```python
from build123d import *

# Parameters (mm, degrees)
CUT_EXTRUDE1_DEPTH      = 4
CUT_EXTRUDE1_DEPTH_BACK = 4
SKETCH2_W               = 41
SKETCH2_H               = 1.5
SKETCH4_W               = 1.2295
SKETCH4_H               = 15
CUT_EXTRUDE2_DEPTH      = 8
CUT_EXTRUDE2_DEPTH_BACK = 8
SKETCH5_W               = 30
SKETCH5_H               = 3.75


with BuildPart() as part:
    # Sketch1 → Revolve1 (revolve)
    with BuildSketch(Plane(origin=(0, 0, 0), x_dir=(0, 0, -1), z_dir=(1, 0, 0)), mode=Mode.PRIVATE) as revolve1_sk:
        Polygon((-4, 8.5), (-3.5, 8), (3.5, 8), (4, 8.5), (4, 14.5), (3.5, 15), (-3.5, 15), (-4, 14.5), align=None)
    revolve(revolve1_sk.sketch.rotate(Axis((0, 0, -4), (0, 0, 1)), 270), axis=Axis((0, 0, -4), (0, 0, 1)))

    # Sketch2 → Cut-Extrude1 (cut, two sides: drawn at the far end of the back side and taken through both)
    with BuildSketch(Plane.XY.offset(-CUT_EXTRUDE1_DEPTH_BACK)):
        with Locations((-9.5, 0)):
            Rectangle(SKETCH2_W, SKETCH2_H)
    extrude(amount=CUT_EXTRUDE1_DEPTH + CUT_EXTRUDE1_DEPTH_BACK, mode=Mode.SUBTRACT)

    # Sketch3 → Cut-Revolve1 (revolve, cut)
    with BuildSketch(Plane.XY, mode=Mode.PRIVATE) as cut_revolve1_sk:
        Polygon((-11.5, -15), (-14.5, -15), (-14.5, -3), (-13.2, -3), (-13.2, 0), (-11.5, 0), align=None)
    revolve(cut_revolve1_sk.sketch.rotate(Axis((-11.5, 0, 0), (0, -1, 0)), 270), axis=Axis((-11.5, 0, 0), (0, -1, 0)), mode=Mode.SUBTRACT)

    # Sketch4 → Cut-Revolve2 (revolve, cut)
    with BuildSketch(Plane.XY, mode=Mode.PRIVATE) as cut_revolve2_sk:
        with Locations((-12.11475, 8.25)):
            Rectangle(SKETCH4_W, SKETCH4_H)
    revolve(cut_revolve2_sk.sketch.rotate(Axis((-11.5, 15.75, 0), (0, -1, 0)), 270), axis=Axis((-11.5, 15.75, 0), (0, -1, 0)), mode=Mode.SUBTRACT)

    # Sketch5 → Cut-Extrude2 (cut, two sides: drawn at the far end of the back side and taken through both)
    with BuildSketch(Plane.XY.offset(-CUT_EXTRUDE2_DEPTH_BACK)):
        with Locations((0, 13.875)):
            Rectangle(SKETCH5_W, SKETCH5_H)
    extrude(amount=CUT_EXTRUDE2_DEPTH + CUT_EXTRUDE2_DEPTH_BACK, mode=Mode.SUBTRACT)

    # Sketch6 → Cut-Revolve3 (revolve, cut)
    with BuildSketch(Plane.XY, mode=Mode.PRIVATE) as cut_revolve3_sk:
        Polygon((-5, 2.333333333), (-6.2295, 2.333333333), (-6.2295, 11.7295), (-6.5, 12), (-5, 12), align=None)
    revolve(cut_revolve3_sk.sketch.rotate(Axis((-5, 12, 0), (0, -1, 0)), 270), axis=Axis((-5, 12, 0), (0, -1, 0)), mode=Mode.SUBTRACT)

    # Sketch7 → Cut-Revolve4 (revolve, cut)
    with BuildSketch(Plane.XY, mode=Mode.PRIVATE) as cut_revolve4_sk:
        Polygon((5, 2.333333333), (3.7705, 2.333333333), (3.7705, 11.7295), (3.5, 12), (5, 12), align=None)
    revolve(cut_revolve4_sk.sketch.rotate(Axis((5, 12, 0), (0, -1, 0)), 270), axis=Axis((5, 12, 0), (0, -1, 0)), mode=Mode.SUBTRACT)


solid = part.part
```
Geometry check sheet. Reference: the model listing, model coordinates, mm. A direction names the side the tool comes from. Give positions to 0.01 mm unless a question says otherwise; leave off trailing zeros. Loops run counter-clockwise (first coordinate to the right, second up) from the corner with the lowest first, then second, coordinate; pieces in that order, holes last. Notation, with made-up numbers: M -3.75,11 L 7.25,11 A29 cw 7.25,38 Z; hole C -0.5,-30 d8. An arc over 180 degrees is marked long. Write item = value, one per line.
(1) Sectioned sample at B-B, the plane z = 0. State how many separate pieces and enclosed holes the cut face has, plus the area to 3 significant figures.
Answer below:
separate_pieces = 5
enclosed_holes = 0
area = 359 mm2
(2) Material ranges on line 1 (X direction, y = 6.25, z = 0); line 2 (X direction, y = 3, z = 0); line 3 (Z direction, x = -11, y = -4.5), recorded low to high. Write a range as [from, to].
Answer below:
line_1 = [-13.64, -12.73], [-10.27, -6.23], [6.23, 13.64]
line_2 = [-14.7, -12.73], [-10.27, -7.42], [7.42, 14.7]
line_3 = [-4, -2.96], [2.96, 4]
(3) Sectioned sample at A-A, the plane x = 0. Record the cut outline in (y, z), plus the area to 4 significant figures.
Answer below:
outline = M -15,-3.5 L -14.5,-4 L -8.5,-4 L -8,-3.5 L -8,3.5 L -8.5,4 L -14.5,4 L -15,3.5 Z; M 8,-3.5 L 8.5,-4 L 12,-4 L 12,4 L 8.5,4 L 8,3.5 Z
area = 87.25 mm2
(4) Gauge pin test, flat ends, axial feed: pin 1 Ø1.5 at (x, z) = (9, -0.5) entering from -Y; pin 2 Ø3 at (y, z) = (-2.5, -0.5) entering from -X; pin 3 Ø3 at (x, z) = (5, 0) entering from -Y. Record the tip position at first contact, or that the pin passes through.
Answer below:
pin_1 = -12.53
pin_2 = -14.97
pin_3 = -14.59
(5) Sectioned sample at D-D, the plane z = 2.5. Record the cut outline in (x, y), plus the area to 3 significant figures.
Answer below:
outline = M -14.98,-0.75 A15 ccw -13.16,-7.2 L -13.16,-3 L -9.84,-3 L -9.84,-11.32 A15 ccw long 9,12 L -9,12 A15 ccw -14.98,0.75 L -7.96,0.75 A8 cw 7.96,0.75 L 11,0.75 L 11,-0.75 L 7.96,-0.75 A8 cw -7.96,-0.75 Z
area = 432 mm2
(6) Release check for a two-part mould opening along X. For faces 1 (the face through (6.666, -13.437, 0.049)), 2 (the face through (-12.71, 7.26, 3.86)), 3 (the face through (6.2, 9.17, -0.27)) record: released by +X, released by -X, zero draft, split by the parting line, or undercut.
Answer below:
face_1 = split by the parting line
face_2 = released by -X
face_3 = undercut
(7) Tool access check on faces 4 (the face through (0.17, 8.14, -3.64)), 5 (the face through (0.169, 8.134, 3.635)), 6 (the face through (-13, 0.75, 0)), 7 (the face through (-12.933, -1.859, 0.914)), 8 (the face through (-6.22, 9.17, -0.16)). Record the directions out of +Z, -Z, +X, -X, +Y, -Y that give a thin tool (end or side, any length) a straight path to the whole face; none if there is none.
Answer below:
face_4 = -Z
face_5 = +Z
face_6 = +Z, -Z, -X
face_7 = -Y
face_8 = +Y
